```python
from build123d import *

# Parameters (mm, degrees)
MODEL_R             = 5
BOSS_EXTRUDE1_DEPTH = 3


with BuildPart() as part:
    # Model → Boss-Extrude1 (new body)
    with BuildSketch(Plane.XY):
        Polygon((352.69017886, 199.123752973), (352.69017886, 169.123752973), (349.69017886, 169.123752973), (349.69017886, 139.123752973), (341.69017886, 139.123752973), (341.69017886, 142.123752973), (331.69017886, 142.123752973), (331.69017886, 139.123752973), (322.69017886, 139.123752973), (322.69017886, 200.123752973), (292.69017886, 200.123752973), (292.69017886, 139.123752973), (270.69017886, 139.123752973), (270.69017886, 142.123752973), (260.69017886, 142.123752973), (260.69017886, 139.123752973), (251.69017886, 139.123752973), (251.69017886, 169.123752973), (254.69017886, 169.123752973), (254.69017886, 199.123752973), (251.69017886, 199.123752973), (251.69017886, 254.123752973), (254.69017886, 254.123752973), (287.684060801, 245.441152462), (286.920580903, 242.539928851), (315.932817021, 234.905129872), (316.696296919, 237.806353484), (349.69017886, 229.123752973), (349.69017886, 199.123752973), align=None)
        with Locations((271.859853833, 239.264952873)):
            Circle(MODEL_R, mode=Mode.SUBTRACT)
    extrude(amount=BOSS_EXTRUDE1_DEPTH)


solid = part.part
```
CAD build for the part. Positions are in the model's coordinates, mm. A direction names the side the tool comes from. Give positions to 0.01 mm unless a question says otherwise; leave off trailing zeros. Write each loop counter-clockwise with the first axis right and the second up, starting at its lowest first coordinate (ties: lowest second). Pieces come first, ordered by that corner, then holes. Notation, with made-up numbers: M 39,-16 L 93,-16 A17 cw 93,-4 Z; hole C 87,68.25 d11. An arc over 180 degrees is marked long. Return JSON: item names as keys, results as strings. Group by question number.
(1) Flat gauge pins, fed straight in: pin 1 Ø0.9 at (x, z) = (336, 1) entering from -Y; pin 2 Ø1.5 at (y, z) = (211.5, 2) entering from +X; pin 3 Ø1 at (y, z) = (189.5, 1.5) entering from -X. Where does each tip first touch, or does it go through?
(2) Drill centre lines: L1, parallel to X at y = 196.5, z = 2.6; L2, parallel to X at y = 156.5, z = 2.85; L3, parallel to X at y = 208.5, z = 2.15. Where is each one in solid material? Low to high. Write a range as [from, to].
(3) Band-saw the part on A-A (y = 176). Give the cut face in (x, z), and give its area (3 significant figures).
(4) 3-axis set-ups, long thin cutter, end or side, ignore diameter. For faces 1 (the face through (349.69, 154, 1)), 2 (the face through (331.69, 141, 1)), 3 (the face through (316.3, 236.3, 1.5)), 4 (the face through (253, 199.124, 1)), 5 (the face through (287.308, 244.011, 1.479)): which of +Z, -Z, +X, -X, +Y, -Y reach the whole face in a straight line?
(5) Mould opens along Y. For faces 6 (the face through (251.69, 154, 1)), 7 (the face through (253, 169.124, 1)), 8 (the face through (332.962, 233.526, 1.479)), 9 (the face through (351, 169.124, 1)) say: pulls with the +Y half, pulls with the -Y half, needs draft (parallel to the pull), parting line crosses it, or undercut.
(6) Band-saw the part on B-B (x = 273). Give the cut face in (y, z).
(7) Band-saw the part on D-D (y = 208). Give the cut face in (x, z).
Entries:
{
 "1": {"pin 1": "stops at y = 142.12", "pin 2": "stops at x = 349.69", "pin 3": "stops at x = 254.69"},
 "2": {"L1": "x = [254.69, 292.69], [322.69, 352.69]", "L2": "x = [251.69, 292.69], [322.69, 349.69]", "L3": "x = [251.69, 349.69]"},
 "3": {"outline": "M 254.69,0 L 292.69,0 L 292.69,3 L 254.69,3 Z; M 322.69,0 L 352.69,0 L 352.69,3 L 322.69,3 Z", "area": "204 mm^2"},
 "4": {"face 1": "+Z, -Z, +X, -Y", "face 2": "+Z, -Z, -Y", "face 3": "+Z, -Z, +Y", "face 4": "+Z, -Z, -X", "face 5": "+Z, -Z, +X"},
 "5": {"face 6": "needs draft", "face 7": "undercut", "face 8": "pulls with the +Y half", "face 9": "pulls with the -Y half"},
 "6": {"outline": "M 139.12,0 L 234.4,0 L 234.4,3 L 139.12,3 Z; M 244.13,0 L 249.31,0 L 249.31,3 L 244.13,3 Z"},
 "7": {"outline": "M 251.69,0 L 349.69,0 L 349.69,3 L 251.69,3 Z"}
}
